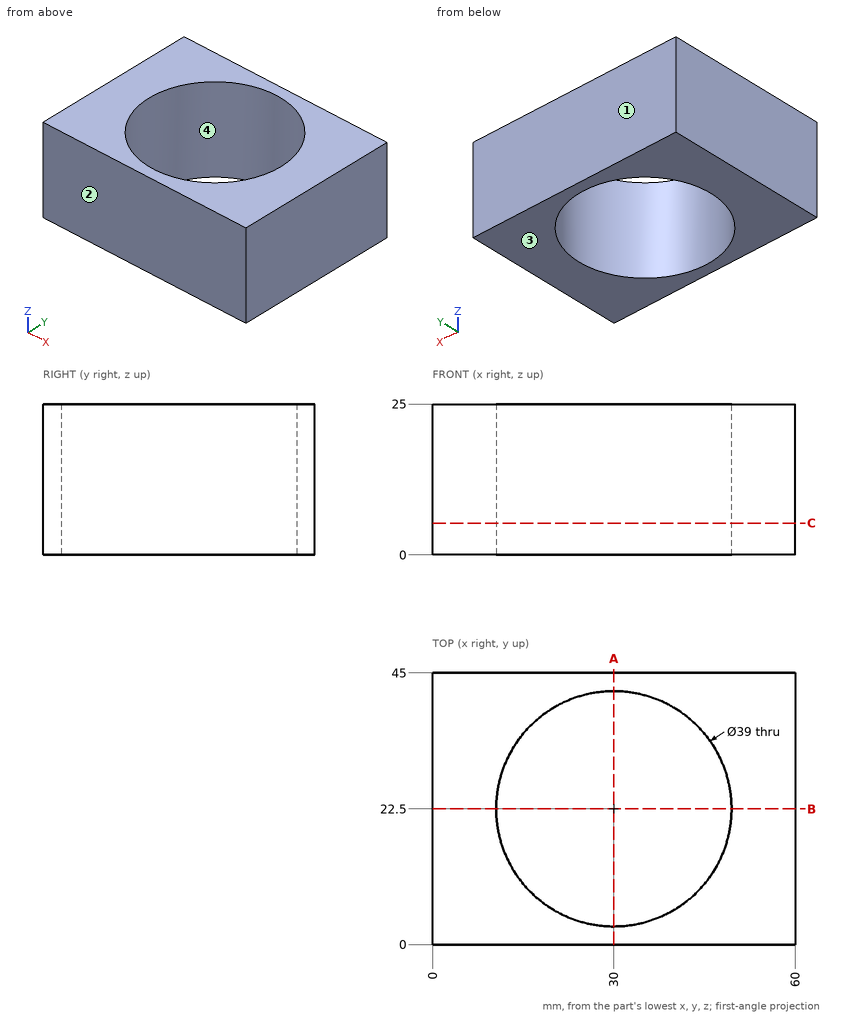
Job drawing, mm, ordinate dimensions from the low corner. One solid piece. Round coordinates to 2 decimals unless told otherwise and drop trailing zeros. Order: outer loops, then holes, each group sorted by start corner. A loop starts at its lowest first (then second) coordinate and runs counter-clockwise, first axis right, second up. Notation, with made-up numbers: (14, -22) -> (56, -22) arc R35 ccw to (56, 13) -> close; hole circle Ø2 at (-22, -36.5). An arc over 180 degrees is marked (long way). Answer in a Markdown table with one row per item.
1) Mould opens along Y. For the marked faces 1, 2, 3 and 4 say: released by +Y, released by -Y, zero draft, split by the parting line, or undercut.
Values:
| item | result |
|---|---|
| face 1 | released by +Y |
| face 2 | released by -Y |
| face 3 | zero draft |
| face 4 | undercut |
2) Band-saw the part on B-B on y = 22.5. Give the cut face in (x, z), and give its area (3 significant figures).
Values:
| item | result |
|---|---|
| outline | (0, 0) -> (10.5, 0) -> (10.5, 25) -> (0, 25) -> close; (49.5, 0) -> (60, 0) -> (60, 25) -> (49.5, 25) -> close |
| area | 525 mm2 |
3) Wall check: L1, parallel to Y at x = 30, z = 9.5; L2, parallel to X at y = 23, z = 9.75; L3, parallel to X at y = 7.5, z = 2.25. Give the ranges that are in metal, low to high.
Values:
| item | result |
|---|---|
| L1 | 0 to 3, 42 to 45 |
| L2 | 0 to 10.51, 49.49 to 60 |
| L3 | 0 to 17.54, 42.46 to 60 |
4) Band-saw the part on A-A on x = 30. Give the cut face in (y, z), and give its area (3 significant figures).
Values:
| item | result |
|---|---|
| outline | (0, 0) -> (3, 0) -> (3, 25) -> (0, 25) -> close; (42, 0) -> (45, 0) -> (45, 25) -> (42, 25) -> close |
| area | 150 mm2 |
5) Band-saw the part on C-C on z = 5.25. Give the cut face in (x, y).
Values:
| item | result |
|---|---|
| outline | (0, 0) -> (60, 0) -> (60, 45) -> (0, 45) -> close; hole circle Ø39 at (30, 22.5) |
